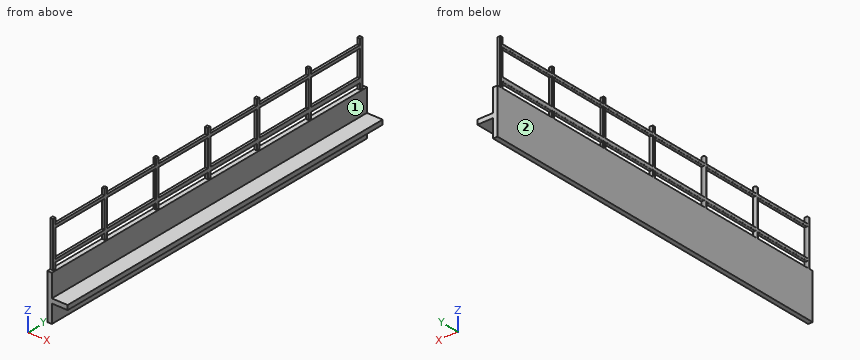
```python
from build123d import *

# Parameters (mm, degrees)
F1_DEPTH = 165
F2_W     = 1.3
F2_H     = 1.3
F3_DEPTH = 20
F4_W     = 25.7
F4_H     = 1.3
F4_W_2   = 24.4
F5_DEPTH = 1.3
F6_R     = 0.3


with BuildPart() as f1:
    # F0 (on Front) → F1 (new body)
    with BuildSketch(Plane.XZ):
        Polygon((7, 0), (0, 0), (0, 10), (-2, 10), (-2, -10), (0, -10), (0, -2), (7, -2), align=None)
    extrude(amount=F1_DEPTH)

    # F2 (on face) → F3 (join)
    with BuildSketch(Plane.XY.offset(10)):
        with Locations((-1.35, -2.15)):
            Rectangle(F2_W, F2_H)
        with Locations((-1.35, -29.15)):
            Rectangle(F2_W, F2_H)
        with Locations((-1.35, -56.15)):
            Rectangle(F2_W, F2_H)
        with Locations((-1.35, -81.85)):
            Rectangle(F2_W, F2_H)
        with Locations((-1.35, -108.85)):
            Rectangle(F2_W, F2_H)
        with Locations((-1.35, -135.85)):
            Rectangle(F2_W, F2_H)
        with Locations((-1.35, -162.85)):
            Rectangle(F2_W, F2_H)
    extrude(amount=F3_DEPTH)

    # F4 (on face) → F5 (join)
    with BuildSketch(Plane(origin=(-2, 0, 0), x_dir=(0, -1, 0), z_dir=(-1, 0, 0))):
        Polygon((2.8, 14.5544293599), (2.8, 12.6), (28.5, 12.6), (28.5, 14.4497695307), align=None)
        with Locations((15.65, 26.75)):
            Rectangle(F4_W, F4_H)
        with Locations((42.65, 26.75)):
            Rectangle(F4_W, F4_H)
        Polygon((29.8, 14.4444754537), (29.8, 12.6), (55.5, 12.6), (55.5, 14.3398156246), align=None)
        with Locations((69, 26.75)):
            Rectangle(F4_W_2, F4_H)
        Polygon((56.8, 14.3345215476), (56.8, 12.6), (81.2, 12.6), (81.2, 14.2351557954), align=None)
        Polygon((82.5, 14.2298617184), (82.5, 12.6), (108.2, 12.6), (108.2, 14.1252018892), align=None)
        with Locations((95.35, 26.75)):
            Rectangle(F4_W, F4_H)
        with Locations((122.35, 26.75)):
            Rectangle(F4_W, F4_H)
        Polygon((109.5, 12.6), (135.2, 12.6), (135.2, 14.0152479831), (109.5, 14.1199078123), align=None)
        Polygon((136.5, 12.6), (162.2, 12.6), (162.2, 13.905294077), (136.5, 14.0099539061), align=None)
        with Locations((149.35, 26.75)):
            Rectangle(F4_W, F4_H)
    extrude(amount=-F5_DEPTH)

    # F6
    f6_edges = [f1.edges().sort_by_distance(p)[0] for p in [
        (-2, -135.2, 11.3),
        (-2, -136.5, 11.3),
        (-2, -149.35, 12.6),
        (-2, -149.35, 13.957624),
        (-2, -162.2, 11.3),
        (-2, -163.5, 20),
        (-2, -162.2, 20.002647),
        (-2, -149.35, 27.4),
        (-2, -149.35, 26.1),
        (-2, -136.5, 20.054977),
        (-2, -136.5, 28.7),
        (-2, -135.2, 28.7),
        (-2, -135.2, 20.057624),
        (-2, -122.35, 14.067578),
        (-2, -122.35, 12.6),
        (-2, -122.35, 26.1),
        (-2, -122.35, 27.4),
        (-2, -162.2, 28.7),
        (-2, -109.5, 28.7),
        (-2, -95.35, 27.4),
        (-2, -95.35, 14.177532),
        (-2, -108.2, 20.112601),
        (-2, -95.35, 12.6),
        (-2, -108.2, 11.3),
        (-2, -82.5, 20.164931),
        (-2, -82.5, 28.7),
        (-2, -69, 27.4),
        (-2, -69, 26.1),
        (-2, -81.2, 20.167578),
        (-2, -69, 14.284839),
        (-2, -69, 12.6),
        (-2, -82.5, 11.3),
        (-2, -81.2, 28.7),
        (-2, -81.2, 11.3),
        (-2, -56.8, 28.7),
        (-2, -56.8, 20.217261),
        (-2, -56.8, 11.3),
        (-2, -42.65, 12.6),
        (-2, -42.65, 14.392146),
        (-2, -55.5, 20.219908),
        (-2, -42.65, 26.1),
        (-2, -42.65, 27.4),
        (-2, -55.5, 28.7),
        (-2, -29.8, 28.7),
        (-2, -15.65, 27.4),
        (-2, -15.65, 26.1),
        (-2, -29.8, 20.272238),
        (-2, -28.5, 20.274885),
        (-2, -29.8, 11.3),
        (-2, -28.5, 28.7),
        (-2, -2.8, 28.7),
        (-2, -1.5, 20),
        (-2, -2.8, 20.327215),
        (-2, -15.65, 14.502099),
        (-2, -15.65, 12.6),
        (-2, -2.8, 11.3),
        (-2, -28.5, 11.3),
        (-2, -55.5, 11.3),
        (-2, -95.35, 26.1),
        (-2, -109.5, 11.3),
        (-2, -109.5, 20.109954),
        (-2, -108.2, 28.7),
    ]]
    fillet(f6_edges, radius=F6_R)


solid = f1.part
```
Geometry check sheet. Reference: the model listing, model coordinates, mm. Face numbers are marked on the shaded views. A direction names the side the tool comes from. Round coordinates to 2 decimals unless told otherwise and drop trailing zeros. Order: outer loops, then holes, each group sorted by start corner. A loop starts at its lowest first (then second) coordinate and runs counter-clockwise, first axis right, second up. Notation, with made-up numbers: M 43,6.25 L 95,6.25 A15 cw 95,29.25 Z; hole C -8,70 d4. An arc over 180 degrees is marked long. Write item = value, one per line.
Q1. Section check C-C (z = 3.5). Enter the section's corners in (x, y).
Answer block:
outline = M -2,-165 L 0,-165 L 0,0 L -2,0 Z
Q2. Depth check by flat-ended pin: pin 1 Ø0.8 at (x, z) = (-1, 20) entering from -Y; pin 2 Ø8 at (y, z) = (-136.5, 15) entering from +X; pin 3 Ø1.1 at (x, z) = (-1, 17.5) entering from +Y; pin 4 Ø4 at (x, z) = (2, 11.5) entering from -Y. Enter the tip coordinate at first touch or a pass-through.
Answer block:
pin_1 = -163.5
pin_2 = -0.7
pin_3 = -1.5
pin_4 = through
Q3. Section check D-D (x = 4.75). Enter the section's corners in (y, z), plus the area to 3 significant figures.
Answer block:
outline = M -165,-2 L 0,-2 L 0,0 L -165,0 Z
area = 330 mm^2
Q4. Set-up check for the marked faces 1 and 2: record each of +Z, -Z, +X, -X, +Y, -Y from which the full face is reachable in a straight line by a thin tool's end or side.
Answer block:
face_1 = +Z, +X, +Y, -Y
face_2 = +Z, -Z, -X, +Y, -Y
Q5. Scan lines: line 1 (Z direction, x = -1, y = -115.5); line 2 (Z direction, x = -1.25, y = -140.5); line 3 (Z direction, x = 6.25, y = -90). Record each from-to range of solid material in increasing order.
Answer block:
line_1 = -10 to 10, 12.6 to 14.1, 26.1 to 27.4
line_2 = -10 to 10, 12.6 to 13.99, 26.1 to 27.4
line_3 = -2 to 0
Q6. Section check A-A (z = 22.5). Give the number of separate pieces and of enclosed holes in the cut face, plus the area to 3 significant figures.
Answer block:
separate_pieces = 7
enclosed_holes = 0
area = 11.6 mm^2
